Part model, mm, in its own coordinate system. A direction names the side the tool comes from. Round coordinates to 2 decimals unless told otherwise and drop trailing zeros. Write each loop counter-clockwise with the first axis right and the second up, starting at its lowest first coordinate (ties: lowest second). Pieces come first, ordered by that corner, then holes. Notation, with made-up numbers: (23, 55) -> (53, 55) arc R26 cw to (53, 79) -> close; hole circle Ø8 at (9, 43.5). An arc over 180 degrees is marked (long way). Use CSV: the item, a comma, the result in double quotes. Start each with the question number.
(1) Drop flat-ended pins along their axis: pin 1 (5.5 mm diameter, centred on x = 6, y = 101, fed in from +Z); pin 2 (1.8 mm diameter, centred on x = 6.5, y = 171.5, fed in from -Z). Give the stop position or say it passes through.
(2) Probe line 1 (Y direction, x = 6.25, z = -9.5); line 2 (X direction, y = 191, z = -0.75); line 3 (Z direction, x = 4.5, y = 103). List the from-to ranges inside material, lowest first. Write a range as [from, to].
(3) Two-plate mould, pull along Y, no slides. Class faces 3 (the flat face through (6, 0, -6)), 4 (the flat face through (6, 28, -8)), 5 (the flat face through (0, 99, -4)), 6 (the flat face through (6, 172, -8)): released by +Y, released by -Y, zero draft, split by the parting line, or undercut.
(4) Saw through at A-A (y = 125). Give the cut face in (x, z), plus the area to 3 significant figures.
(5) Saw through at B-B (x = 4.75). Give the cut face in (y, z).
(6) Which spindle directions (+Z, -Z, +X, -X, +Y, -Y) get a long thin tool onto all of the face, cutting with end or side? Do faces 1 (the flat face through (6, 99, -3)), 2 (the flat face through (6, 200, -6)). Say none if no direction does.
```python
from build123d import *

# Parameters (mm, degrees)
BOSS_EXTRUDE1_DEPTH = 200
SKETCH2_W           = 12.48
SKETCH2_H           = 6
CUT_EXTRUDE1_DEPTH  = 2
CUT_EXTRUDE2_DEPTH  = 201
FILLET1_R           = 0.5


with BuildPart() as part:
    # Sketch1 → Boss-Extrude1 (new body)
    with BuildSketch(Plane(origin=(0, 0, 0), x_dir=(1, 0, 0), z_dir=(0, 1, 0))):
        with BuildLine():
            Line((0, 8), (2, 10))
            Line((2, 10), (10.48, 10))
            Line((10.48, 10), (12.48, 8))
            Line((12.48, 8), (12.48, 1))
            ThreePointArc((12.48, 1), (12.187106781, 0.292893219), (11.48, 0))
            Line((11.48, 0), (1, 0))
            ThreePointArc((1, 0), (0.292893219, 0.292893219), (0, 1))
            Line((0, 1), (0, 8))
        make_face()
    extrude(amount=BOSS_EXTRUDE1_DEPTH)

    # Sketch2 → Cut-Extrude1 (cut)
    with BuildSketch(Plane(origin=(0, 0, -10), x_dir=(-1, 0, 0), z_dir=(0, 0, -1))):
        with Locations((-6.24, 172)):
            Rectangle(SKETCH2_W, SKETCH2_H)
        with Locations((-6.24, 28)):
            Rectangle(SKETCH2_W, SKETCH2_H)
    extrude(amount=-CUT_EXTRUDE1_DEPTH, mode=Mode.SUBTRACT)

    # Sketch3 → Cut-Extrude2 (cut, through all)
    with BuildSketch(Plane.XZ):
        Polygon((1.79, 0), (1.79, -2), (2.79, -3), (9.69, -3), (10.69, -2), (10.69, 0), align=None)
    extrude(amount=-CUT_EXTRUDE2_DEPTH, mode=Mode.SUBTRACT)

    # Fillet1
    fillet1_edges = [part.edges().sort_by_distance(p)[0] for p in [
        (1.79, 100, 0),
        (10.69, 100, 0),
    ]]
    fillet(fillet1_edges, radius=FILLET1_R)


solid = part.part
```
Answers:
1,pin 1,"stops at z = -3"
1,pin 2,"stops at z = -8"
2,line 1,"y = [0, 25], [31, 169], [175, 200]"
2,line 2,"x = [0.03, 1.79], [10.69, 12.45]"
2,line 3,"z = [-10, -3]"
3,face 3,"released by -Y"
3,face 4,"undercut"
3,face 5,"zero draft"
3,face 6,"undercut"
4,outline,"(0, -8) -> (2, -10) -> (10.48, -10) -> (12.48, -8) -> (12.48, -1) arc R1 ccw to (11.48, 0) -> (11.19, 0) arc R0.5 ccw to (10.69, -0.5) -> (10.69, -2) -> (9.69, -3) -> (2.79, -3) -> (1.79, -2) -> (1.79, -0.5) arc R0.5 ccw to (1.29, 0) -> (1, 0) arc R1 ccw to (0, -1) -> close"
4,area,"94.6 mm²"
5,outline,"(0, -10) -> (25, -10) -> (25, -8) -> (31, -8) -> (31, -10) -> (169, -10) -> (169, -8) -> (175, -8) -> (175, -10) -> (200, -10) -> (200, -3) -> (0, -3) -> close"
6,face 1,"+Z, +Y, -Y"
6,face 2,"+Z, -Z, +X, -X, +Y"
